The listing builds one solid part. Answer for the finished solid, in the listing's coordinates (mm). A direction names the side the tool comes from. Coordinates: 2 decimals unless noted, no trailing zeros. Loops run counter-clockwise (first coordinate to the right, second up) from the corner with the lowest first, then second, coordinate; pieces in that order, holes last. Notation, with made-up numbers: M 64.5,3 L 106.5,3 A20 ccw 106.5,31 Z; hole C 73.5,76 d9. An arc over 180 degrees is marked long. Answer as a JSON object with one key per item and string values. Group by question number.
1. Determine the mould class of faces 5 (the face through (1, 31, 9.525)), 6 (the face through (22.892, 13, 18)), 7 (the face through (60.992, 0, 40)) for opening direction X: released by +X, released by -X, zero draft, split by the parting line, or undercut.
2. Straight lines are drawn through the part: L1, parallel to Y at x = 24, z = 17; L2, parallel to X at y = 1.5, z = 25; L3, parallel to Y at x = 11.5, z = 50.5 (3 decimals). For each, find the intervals that lie inside material, in ascending order.
3. A cutting plane is placed at A-A on y = 39.5. Give the vertices of the cut face in (x, z) (3 decimals), and give its area (3 significant figures).
4. A cutting plane is placed at B-B on x = 93. Give the vertices of the cut face in (y, z) (3 decimals).
5. For faces 1 (the face through (41.942, -1, 4)), 2 (the face through (3, -15.875, 30)), 3 (the face through (3, 0, 30)), 4 (the face through (67, -25.4, 45)), determine the directions among +Z, -Z, +X, -X, +Y, -Y from which every point of the face is accessible in a straight line to the end or side of a thin tool.
6. Given pin 1 (5 mm diameter, centred on x = 75, z = 49.5, fed in from +Y); pin 2 (24 mm diameter, centred on x = 20.5, y = -50.5, fed in from +Z) (3 decimals); pin 3 (2.5 mm diameter, centred on y = -8.5, z = 40.5, fed in from -X), each flat-ended and moving along its own axis, determine where each tip first touches the part or whether it passes through.
from build123d import *

# Parameters (mm, degrees)
F1_DEPTH = 63.5
F0_W     = 25.4
F0_H     = 4.7752
F0_H_2   = 4.7498
F0_H_3   = 19.05
F2_DEPTH = 25.4
F3_DEPTH = 15.875


with BuildPart() as f1:
    # F0 (on Front) → F1 (new body, symmetric)
    with BuildSketch(Plane.XZ):
        Polygon((-41.9416204095, -9.525), (41.9416204095, -9.525), (41.9416204095, 9.525), (22.8916204095, 9.525), (-41.9416204095, 9.525), align=None)
    extrude(amount=F1_DEPTH, both=True)

    # F0 (on Front) → F2 (join, symmetric)
    with BuildSketch(Plane.XZ):
        with BuildLine():
            Line((22.8916204095, 9.525), (41.9416204095, 9.525))
            Line((41.9416204095, 9.525), (41.9416204095, 27.0002))
            ThreePointArc((41.9416204095, 27.0002), (46.5913002582, 38.2255201513), (57.8166204095, 42.8752))
            Line((57.8166204095, 42.8752), (60.9916204095, 42.8752))
            Line((60.9916204095, 42.8752), (60.9916204095, 61.9252))
            Line((60.9916204095, 61.9252), (57.8166204095, 61.9252))
            add(Edge.make_bspline(
                [(47.6262813731, 60.4054782554), (50.8985735157, 60.9424204342), (54.2930453114, 61.4486153253), (57.8166204095, 61.9252)],
                knots=[105.8157704089, 105.8157704089, 105.8157704089, 105.8157704089, 112.6831290448, 112.6831290448, 112.6831290448, 112.6831290448], degree=3))
            ThreePointArc((47.6262813731, 60.4054782554), (29.7483713026, 47.7831020369), (22.8916204095, 27.0002))
            Line((22.8916204095, 27.0002), (22.8916204095, 9.525))
        make_face()
        with Locations((73.6916204095, 40.4876)):
            Rectangle(F0_W, F0_H)
        with Locations((73.6916204095, 64.3001)):
            Rectangle(F0_W, F0_H_2)
        with Locations((73.6916204095, 52.4002)):
            Rectangle(F0_W, F0_H_3)
        Polygon((86.3916204095, 61.9252), (86.3916204095, 42.8752), (86.3916204095, 38.1), (111.7916204095, 38.1), (111.7916204095, 66.675), (86.3916204095, 66.675), align=None)
    extrude(amount=F2_DEPTH, both=True)

    # F0 (on Front) → F3 (join)
    with BuildSketch(Plane.XZ):
        with BuildLine():
            add(Edge.make_bspline(
                [(-41.9416204095, 9.525), (-24.2078539178, 36.5584305008), (-2.7948677813, 52.1319988404), (47.6262813731, 60.4054782554)],
                knots=[0, 0, 0, 0, 105.8157704089, 105.8157704089, 105.8157704089, 105.8157704089], degree=3))
            Line((-41.9416204095, 9.525), (22.8916204095, 9.525))
            Line((22.8916204095, 9.525), (22.8916204095, 27.0002))
            ThreePointArc((22.8916204095, 27.0002), (29.7483713026, 47.7831020369), (47.6262813731, 60.4054782554))
        make_face()
    extrude(amount=F3_DEPTH)


solid = f1.part
From the geometry:
{
 "1": {"face 5": "zero draft", "face 6": "released by -X", "face 7": "undercut"},
 "2": {"L1": "y = -25.4 to 25.4", "L2": "x = 22.89 to 41.94", "L3": "y = -15.875 to 0"},
 "3": {"outline": "M -41.942,-9.525 L 41.942,-9.525 L 41.942,9.525 L -41.942,9.525 Z", "area": "1,600 mm²"},
 "4": {"outline": "M -25.4,38.1 L 25.4,38.1 L 25.4,66.675 L -25.4,66.675 Z"},
 "5": {"face 1": "-Z, +X, +Y, -Y", "face 2": "+Z, -X, -Y", "face 3": "+Z, -X, +Y", "face 4": "+Z, +X, -X, -Y"},
 "6": {"pin 1": "stops at y = 25.4", "pin 2": "stops at z = 9.525", "pin 3": "stops at x = -13.74"}
}
